Build history of the part. All positions in model axes, mm. A direction names the side the tool comes from. Round coordinates to 2 decimals unless told otherwise and drop trailing zeros. Write each loop counter-clockwise with the first axis right and the second up, starting at its lowest first coordinate (ties: lowest second). Pieces come first, ordered by that corner, then holes. Notation, with made-up numbers: (59, -6.75) - (83, -6.75) arc R16 ccw to (83, 3.25) - close; hole circle Ø6 at (-1, 49). An arc over 180 degrees is marked (long way). Answer as a JSON object with one key per item and string values. Group by question number.
Item 1: Slice it at D-D, the plane x = 36.5. List the corners of the cut face in (y, z).
Item 2: Which spindle directions (+Z, -Z, +X, -X, +Y, -Y) get a long thin tool onto all of the face, cutting with end or side? Do faces 4 (the flat face through (30.125, 37.447, -57.159)), 5 (the flat face through (-26.5, 0, -36)), 6 (the flat face through (30, 40, -59)), 7 (the flat face through (35.352, -21.584, -36.482)). Say none if no direction does.
Item 3: Slice it at C-C, the plane y = 12.5. List the corners of the cut face in (x, z).
Item 4: Probe line 1 (X direction, y = 33.5, z = -38.5); line 2 (Z direction, x = 31, y = -47.5); line 3 (X direction, y = -1, z = -40). List the from-to ranges inside material, lowest first. Write a range as from..to.
Item 5: Flat gauge pins, fed straight in: pin 1 (2 mm diameter, centred on x = -10, y = 35, fed in from +Z); pin 2 (6 mm diameter, centred on y = 10.5, z = -50.5, fed in from +X); pin 3 (4 mm diameter, centred on x = 30.5, z = -65, fed in from +Y). Where does each tip first touch, or does it go through?
Item 6: Slice it at B-B, the plane z = -20.5. List the corners of the cut face in (x, y).
Item 7: Two-plate mould, pull along X, no slides. Class faces 1 (the flat face through (-42.5, 35, -58)), 2 (the flat face through (-1, 1, -74)), 3 (the flat face through (41, -35, -57)): +X half, -X half, draft (parallel to the pull), parting line (faces both ways), or undercut.
from build123d import *

# Parameters (mm, degrees)
F1_DEPTH = 74
F3_DEPTH = 50
F4_T     = -1.5


with BuildPart() as f1:
    # F0 (on Top) → F1 (new body)
    with BuildSketch(Plane.XY):
        Polygon((42.5, 27.5), (42.5, 52.5), (-42.5, 52.5), (-42.5, 27.5), (-28, 15.5), (-28, -15.5), (-42.5, -27.5), (-42.5, -52.5), (42.5, -52.5), (42.5, -27.5), (28, -15.5), (28, 15.5), (29, 16.3275862069), align=None)
        with BuildLine():
            Line((-34.6619805153, -37.7418373828), (-29.712233047, -32.7920899145))
            ThreePointArc((-29.712233047, -32.7920899145), (-23.3482720164, -32.7920899145), (-23.3482720164, -39.1560509451))
            Line((-23.3482720164, -39.1560509451), (-28.2980194847, -44.1057984134))
            ThreePointArc((-28.2980194847, -44.1057984134), (-34.6619805153, -44.1057984134), (-34.6619805153, -37.7418373828))
        make_face(mode=Mode.SUBTRACT)
        with BuildLine():
            ThreePointArc((34.6619805153, -37.7418373828), (34.6619805153, -44.1057984134), (28.2980194847, -44.1057984134))
            Line((28.2980194847, -44.1057984134), (23.3482720164, -39.1560509451))
            ThreePointArc((23.3482720164, -39.1560509451), (23.3482720164, -32.7920899145), (29.712233047, -32.7920899145))
            Line((29.712233047, -32.7920899145), (34.6619805153, -37.7418373828))
        make_face(mode=Mode.SUBTRACT)
        with BuildLine():
            ThreePointArc((-34.6619805153, 37.7418373828), (-34.6619805153, 44.1057984134), (-28.2980194847, 44.1057984134))
            Line((-28.2980194847, 44.1057984134), (-23.3482720164, 39.1560509451))
            ThreePointArc((-23.3482720164, 39.1560509451), (-23.3482720164, 32.7920899145), (-29.712233047, 32.7920899145))
            Line((-29.712233047, 32.7920899145), (-34.6619805153, 37.7418373828))
        make_face(mode=Mode.SUBTRACT)
        with BuildLine():
            ThreePointArc((29.712233047, 32.7920899145), (29.3709433721, 32.4840166266), (29, 32.2123756731))
            ThreePointArc((29, 32.2123756731), (23.3244813451, 32.8160598061), (22.8060506298, 38.5))
            ThreePointArc((22.8060506298, 38.5), (23.0616159687, 38.8408735961), (23.3482720164, 39.1560509451))
            Line((23.3482720164, 39.1560509451), (28.2980194847, 44.1057984134))
            ThreePointArc((28.2980194847, 44.1057984134), (28.6345514487, 44.4099938176), (29, 44.6787613065))
            ThreePointArc((29, 44.6787613065), (34.6382034894, 44.1293990809), (35.2714518059, 38.5))
            ThreePointArc((35.2714518059, 38.5), (34.9872627822, 38.1044016861), (34.6619805153, 37.7418373828))
            Line((34.6619805153, 37.7418373828), (29.712233047, 32.7920899145))
        make_face(mode=Mode.SUBTRACT)
        with BuildLine():
            Line((23.3482720164, -39.1560509451), (28.2980194847, -44.1057984134))
            ThreePointArc((28.2980194847, -44.1057984134), (34.6619805153, -44.1057984134), (34.6619805153, -37.7418373828))
            Line((34.6619805153, -37.7418373828), (29.712233047, -32.7920899145))
            ThreePointArc((29.712233047, -32.7920899145), (23.3482720164, -32.7920899145), (23.3482720164, -39.1560509451))
        make_face()
        with BuildLine():
            Line((-23.3482720164, 39.1560509451), (-28.2980194847, 44.1057984134))
            ThreePointArc((-28.2980194847, 44.1057984134), (-34.6619805153, 44.1057984134), (-34.6619805153, 37.7418373828))
            Line((-34.6619805153, 37.7418373828), (-29.712233047, 32.7920899145))
            ThreePointArc((-29.712233047, 32.7920899145), (-23.3482720164, 32.7920899145), (-23.3482720164, 39.1560509451))
        make_face()
        with BuildLine():
            ThreePointArc((-23.3482720164, -39.1560509451), (-23.3482720164, -32.7920899145), (-29.712233047, -32.7920899145))
            Line((-29.712233047, -32.7920899145), (-34.6619805153, -37.7418373828))
            ThreePointArc((-34.6619805153, -37.7418373828), (-34.6619805153, -44.1057984134), (-28.2980194847, -44.1057984134))
            Line((-28.2980194847, -44.1057984134), (-23.3482720164, -39.1560509451))
        make_face()
        with BuildLine():
            Line((29, 38.4438178981), (29, 32.2123756731))
            ThreePointArc((29, 32.2123756731), (29.3709433721, 32.4840166266), (29.712233047, 32.7920899145))
            Line((29.712233047, 32.7920899145), (34.6619805153, 37.7418373828))
            ThreePointArc((34.6619805153, 37.7418373828), (34.9872627822, 38.1044016861), (35.2714518059, 38.5))
            Line((35.2714518059, 38.5), (29.0561821019, 38.5))
            Line((29.0561821019, 38.5), (29, 38.4438178981))
        make_face()
        with BuildLine():
            ThreePointArc((22.8060506298, 38.5), (23.3244813451, 32.8160598061), (29, 32.2123756731))
            Line((29, 32.2123756731), (29, 38.4438178981))
            Line((29, 38.4438178981), (29, 38.5))
            Line((29, 38.5), (22.8060506298, 38.5))
        make_face()
        with BuildLine():
            Line((29, 38.5), (29.0561821019, 38.5))
            Line((29.0561821019, 38.5), (35.2714518059, 38.5))
            ThreePointArc((35.2714518059, 38.5), (34.6382034894, 44.1293990809), (29, 44.6787613065))
            Line((29, 44.6787613065), (29, 38.5))
        make_face()
        with BuildLine():
            ThreePointArc((23.3482720164, 39.1560509451), (23.0616159687, 38.8408735961), (22.8060506298, 38.5))
            Line((22.8060506298, 38.5), (29, 38.5))
            Line((29, 38.5), (29, 44.6787613065))
            ThreePointArc((29, 44.6787613065), (28.6345514487, 44.4099938176), (28.2980194847, 44.1057984134))
            Line((28.2980194847, 44.1057984134), (23.3482720164, 39.1560509451))
        make_face()
    extrude(amount=-F1_DEPTH)

    # F2 (on Right) → F3 (cut, symmetric)
    with BuildSketch(Plane.YZ):
        Polygon((-52.5, 0), (-52.5, -74), (-20, 0), align=None)
        Polygon((52.8937540948, 0), (20, 0), (52.5, -74), align=None)
    extrude(amount=F3_DEPTH, both=True, mode=Mode.SUBTRACT)

    # F4
    f4_openings = [f1.faces().sort_by_distance(p)[0] for p in [
        (0, 0, 0),
        (0, -36.59684, -37.789727),
        (-1.7e-05, 36.596839, -37.789725),
    ]]
    offset(amount=F4_T, openings=f4_openings, kind=Kind.INTERSECTION)


solid = f1.part
Geometry says:
{
 "1": {"outline": "(-52.5, -74) - (-22.53, -74) - (-22.53, -5.77) - (-24.48, -10.2) - (-24.48, -72.5) - (-51.84, -72.5) - close; (22.53, -74) - (52.5, -74) - (51.84, -72.5) - (24.48, -72.5) - (24.48, -10.2) - (22.53, -5.77) - close"},
 "2": {"face 4": "+Z", "face 5": "+Z, +Y, -Y", "face 6": "+Z, +Y", "face 7": "+Z, -Z, +X"},
 "3": {"outline": "(-28, -74) - (28, -74) - (28, 0) - (26.5, 0) - (26.5, -72.5) - (-26.5, -72.5) - (-26.5, 0) - (-28, 0) - close"},
 "4": {"line 1": "x = -42.5..-41, 41..42.5", "line 2": "z = -74..-72.5", "line 3": "x = -28..-26.5, 26.5..28"},
 "5": {"pin 1": "stops at z = -72.5", "pin 2": "stops at x = 28", "pin 3": "stops at y = 40"},
 "6": {"outline": "(-42.5, -29) - (-41, -29) - (-41, -28.21) - (-26.5, -16.21) - (-26.5, 16.21) - (-41, 28.21) - (-41, 29) - (-42.5, 29) - (-42.5, 27.5) - (-28, 15.5) - (-28, -15.5) - (-42.5, -27.5) - close; (26.5, -16.21) - (41, -28.21) - (41, -29) - (42.5, -29) - (42.5, -27.5) - (28, -15.5) - (28, 15.5) - (42.5, 27.5) - (42.5, 29) - (41, 29) - (41, 28.21) - (26.5, 16.21) - close"},
 "7": {"face 1": "-X half", "face 2": "draft", "face 3": "undercut"}
}
